Input: part model. Units: mm. Frame: model coordinates. Face numbers are marked on the shaded views. A direction names the side the tool comes from. Give positions to 0.01 mm unless a question says otherwise; leave off trailing zeros. Loops run counter-clockwise (first coordinate to the right, second up) from the corner with the lowest first, then second, coordinate; pieces in that order, holes last. Notation, with made-up numbers: (23, 42) -> (66, 42) arc R31 cw to (66, 80) -> close; hole circle Ø10 at (-14.5, -38.75). An arc over 180 degrees is marked (long way). Answer as a JSON object with one key per item and string values.
```python
from build123d import *

# Parameters (mm, degrees)
F0_W     = 96.895166
F0_H     = 51.89516
F1_DEPTH = 25
F2_W     = 60.604836
F2_H     = 28.669358
F3_DEPTH = 25
F4_W     = 19.05242
F4_H     = 12.520161
F4_W_2   = 24.133065
F4_H_2   = 16.875
F5_DEPTH = 66.2


with BuildPart() as f1:
    # F0 (on Front) → F1 (new body)
    with BuildSketch(Plane.XZ):
        Rectangle(F0_W, F0_H)
    extrude(amount=F1_DEPTH)

    # F2 (on Front) → F3 (join)
    with BuildSketch(Plane.XZ):
        Rectangle(F2_W, F2_H)
    extrude(amount=-F3_DEPTH)

    # F4 (on face) → F5 (join)
    with BuildSketch(Plane.XZ.offset(25)):
        with Locations((-16.421372, -0.272178)):
            Rectangle(F4_W, F4_H)
        with Locations((25.856855, -2.268145)):
            Rectangle(F4_W_2, F4_H_2)
    extrude(amount=-F5_DEPTH)

    # F6 (on Top) → F7 (revolve)
    with BuildSketch(Plane.XY):
        with BuildLine():
            Line((-19.05242, 25.040325), (19.596776, 25.040325))
            ThreePointArc((19.596776, 25.040325), (0.272178, 37.411746), (-19.05242, 25.040325))
        make_face()
    revolve(axis=Axis((-1.814518, 0, 0), (1, 0, 0)))


solid = f1.part
```
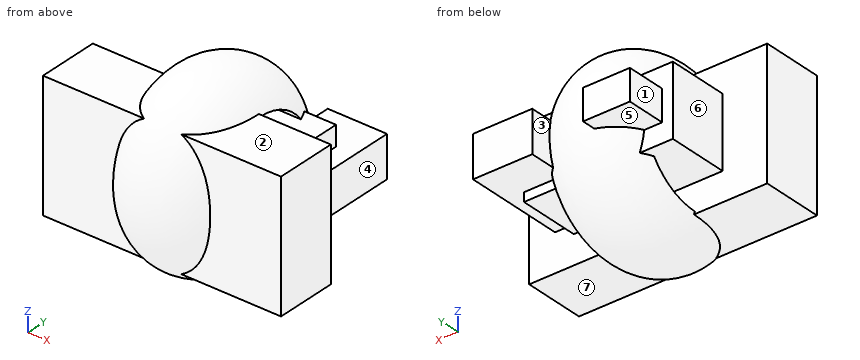
Q1. Pin query (flat end, axial travel): pin 1 (6 mm diameter, centred on x = 36.5, z = 6.5, fed in from -Y); pin 2 (10 mm diameter, centred on y = 37, z = 0, fed in from -X); pin 3 (8 mm diameter, centred on x = 9.5, z = -3, fed in from -Y). Return the tip coordinate at first contact, or that it passes through.
Evaluation:
{"pin 1": "stops at y = -25", "pin 2": "stops at x = -25.95", "pin 3": "stops at y = -36.67"}
Q2. Section A-A, the plane x = 23. Return the cut outline in (y, z), then the cut area to 3 significant figures.
Evaluation:
{"outline": "(-25, -25.95) -> (0, -25.95) -> (0, -14.33) -> (25, -14.33) -> (25, -10.71) -> (41.2, -10.71) -> (41.2, 6.17) -> (25, 6.17) -> (25, 14.33) -> (0, 14.33) -> (0, 25.95) -> (-25, 25.95) -> close", "area": "2,290 mm2"}
Q3. Ray query, line 1 along Z through (x, y) = (-2.5, 7.5); line 2 along Z through (x, y) = (-18.5, 6); line 3 along Z through (x, y) = (23, 23.5). Return the intervals inside material, ascending.
Evaluation:
{"line 1": "z = -36.47 to -23.89, -14.33 to 14.33, 23.89 to 36.47", "line 2": "z = -25.45 to -24.31, -14.33 to 14.33, 24.31 to 25.45", "line 3": "z = -14.33 to 14.33"}
Q4. Section B-B, the plane y = 6. Give the number of separate pieces and of enclosed holes in the cut face, then the cut area to 3 significant figures.
Evaluation:
{"separate pieces": "3", "enclosed holes": "0", "area": "2,570 mm2"}
Q5. Access query for the marked faces 4, 5, 6 and 7. Directions: +Z, -Z, +X, -X, +Y, -Y. A direction counts if a zero-diameter tool reaches every point of the face in a straight line with its end or side. Return the directions, or none.
Evaluation:
{"face 4": "+Z, -Z, +X, +Y", "face 5": "-Z, -X, +Y", "face 6": "+Z, -Z, -X, +Y", "face 7": "-Z, +X, -Y"}
Q6. Draft query along X for the marked faces 1, 2 and 3. Return one class per face: +X half, -X half, draft (parallel to the pull), parting line (faces both ways), or undercut.
Evaluation:
{"face 1": "-X half", "face 2": "draft", "face 3": "undercut"}
